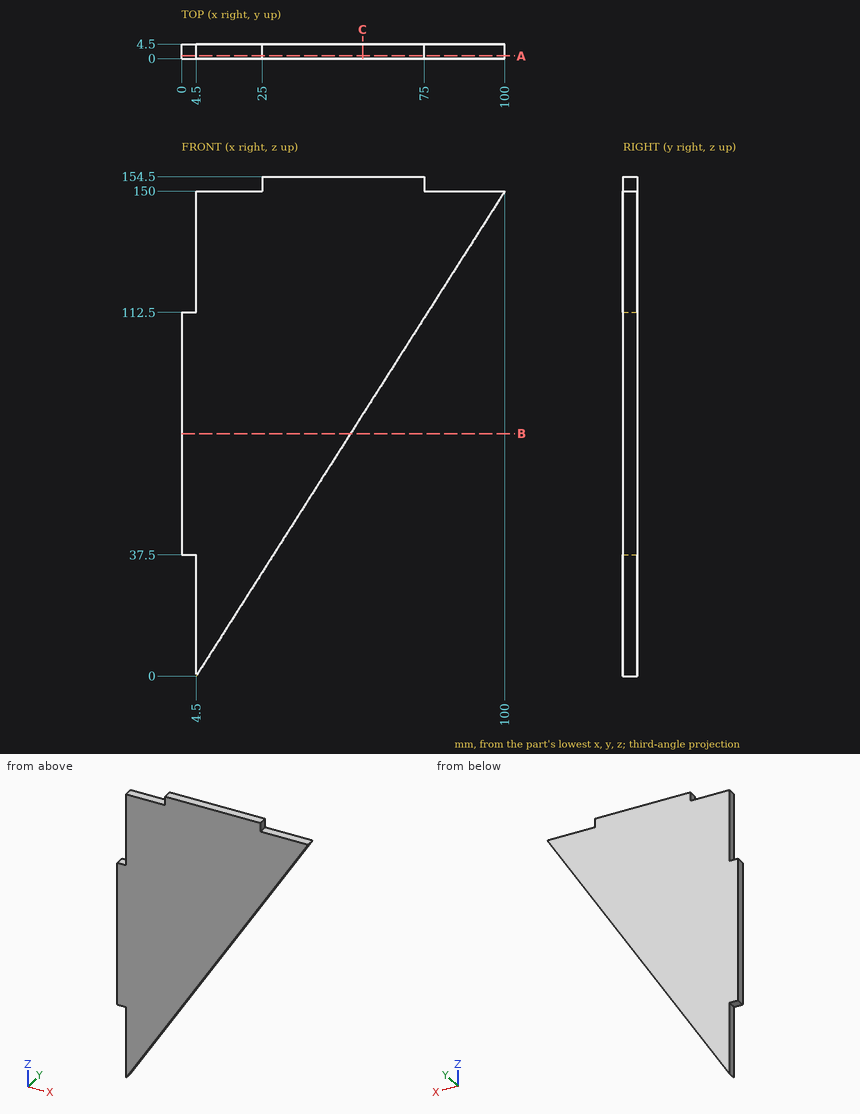
Could you check a few things on this drawing? It's one solid part, dimensions in mm from its lowest x, y, z. Give positions to 0.01 mm unless a question says otherwise; leave off trailing zeros. Write each loop counter-clockwise with the first axis right and the second up, starting at its lowest first coordinate (ties: lowest second). Pieces come first, ordered by that corner, then holes. Notation, with made-up numbers: (-22.75, 83) -> (31.25, 83) arc R19 ccw to (31.25, 118) -> close; hole circle Ø4 at (64.25, 12). An arc over 180 degrees is marked (long way). Write each question's results on one line, items separated by ' | '.
1. Will these pins go through, and if not, where does the flat tip stop? pin 1 Ø1.3 at (x, y) = (14.5, 1.5) entering from +Z; pin 2 Ø1.3 at (y, z) = (3.5, 23) entering from -X; pin 3 Ø1.3 at (y, z) = (2, 152.5) entering from +X.
Check sheet entries:
pin 1: stops at z = 150 | pin 2: stops at x = 4.5 | pin 3: stops at x = 75
2. I need wall thicknesses on L1, parallel to Z at x = 69, y = 3.85; L2, parallel to X at y = 1.55, z = 49; L3, parallel to Z at x = 65, y = 1.2. Which ranges of each line are inside material? Lowest first, please.
Check sheet entries:
L1: z = 101.31 to 154.5 | L2: x = 0 to 35.7 | L3: z = 95.03 to 154.5
3. I want a section at A-A, the plane y = 0.8. Write out the boundary of the cut face in (x, z).
Check sheet entries:
outline: (0, 37.5) -> (4.5, 37.5) -> (4.5, 0) -> (100, 150) -> (75, 150) -> (75, 154.5) -> (25, 154.5) -> (25, 150) -> (4.5, 150) -> (4.5, 112.5) -> (0, 112.5) -> close
4. I want a section at C-C, the plane x = 56. Write out the boundary of the cut face in (y, z).
Check sheet entries:
outline: (0, 80.89) -> (4.5, 80.89) -> (4.5, 154.5) -> (0, 154.5) -> close
5. I want a section at B-B, the plane z = 75. Write out the boundary of the cut face in (x, y).
Check sheet entries:
outline: (0, 0) -> (52.25, 0) -> (52.25, 4.5) -> (0, 4.5) -> close
